Geometry check sheet. Reference: the model listing, model coordinates, mm. A direction names the side the tool comes from. Give positions to 0.01 mm unless a question says otherwise; leave off trailing zeros. Write each loop counter-clockwise with the first axis right and the second up, starting at its lowest first coordinate (ties: lowest second). Pieces come first, ordered by that corner, then holes. Notation, with made-up numbers: M -39.5,41.25 L -26.5,41.25 A18 cw -26.5,50.25 Z; hole C 64,44.5 d5. An arc over 180 degrees is marked long. One line per item, written item: value. Start each with the question number.
1. Cross-section at A-A on z = 0.6. Record the cut outline in (x, y), then the cut area to 3 significant figures.
2. Tool access check on faces 4 (the face through (6.7, 9.04, 2.96)), 5 (the face through (12, 3.25, 3)), 6 (the face through (4, -5, 5)). Record the directions out of +Z, -Z, +X, -X, +Y, -Y that give a thin tool (end or side, any length) a straight path to the whole face; none if there is none.
3. Release check for a two-part mould opening along Y. For faces 1 (the face through (0, -2, 1)), 2 (the face through (13, 4.23, 2.96)), 3 (the face through (-4.285, -10.949, 5.26)) record: pulls with the +Y half, pulls with the -Y half, needs draft (parallel to the pull), parting line crosses it, or undercut.
4. Cross-section at D-D on x = -5.75. Record the cut outline in (y, z), then the cut area to 3 significant figures.
5. Cross-section at B-B on y = -5.25. Record the cut outline in (x, z).
6. Cross-section at C-C on z = 1.9. Record the cut outline in (x, y), then the cut area to 3 significant figures.
7. Gauge pin test, flat ends, axial feed: pin 1 (1.6 mm diameter, centred on y = -7, z = 5.5, fed in from +X); pin 2 (1.5 mm diameter, centred on x = -2, z = 2.5, fed in from +Y); pin 3 (1.2 mm diameter, centred on x = -12, z = 2.5, fed in from -Y). Record the tip position at first contact, or that the pin passes through.
8. Scan lines: line 1 (Y direction, x = 0, z = 0.4); line 2 (Z direction, x = 11, y = -1.25); line 3 (Z direction, x = -1.5, y = -9.5). Record each from-to range of solid material in increasing order.
from build123d import *

# Parameters (mm, degrees)
F1_DEPTH  = 6
F2_T      = -1.5
F3_DEPTH  = 5
F4_T      = -1.5
F5_W      = 25.7072905079
F5_H      = 3
F6_DEPTH  = 14.5
F8_DEPTH  = 2
F9_R      = 2
F10_DEPTH = 25
F11_R     = 1
F12_R     = 1.5
F13_DEPTH = 2


with BuildPart() as f1:
    # F0 (on Top) → F1 (new body)
    with BuildSketch(Plane.XY):
        Polygon((8.1736034401, -11.25), (13.2251681766, 4.2971176266), (0, 13.9057647469), (-13.2251681766, 4.2971176266), (-8.1736034401, -11.25), align=None)
    extrude(amount=F1_DEPTH)

    # F2
    f2_openings = [f1.faces().sort_by_distance(p)[0] for p in [
        (10.699386, -3.476441, 3),
    ]]
    offset(amount=F2_T, openings=f2_openings)

    # F0 (on Top) → F3 (join)
    with BuildSketch(Plane.XY):
        Polygon((8.1736034401, -11.25), (13.2251681766, 4.2971176266), (0, 13.9057647469), (-13.2251681766, 4.2971176266), (-8.1736034401, -11.25), align=None)
    extrude(amount=F3_DEPTH)

    # F4
    f4_openings = [f1.faces().sort_by_distance(p)[0] for p in [
        (0, -11.25, 3),
    ]]
    offset(amount=F4_T, openings=f4_openings)

    # F5 (on face) → F6 (cut)
    with BuildSketch(Plane.XZ.offset(11.25)):
        with Locations((-0.012323726, 3)):
            Rectangle(F5_W, F5_H)
    extrude(amount=-F6_DEPTH, mode=Mode.SUBTRACT)

    # F7 (on face) → F8 (cut)
    with BuildSketch(Plane.XY.offset(6)):
        with BuildLine():
            Line((4, -12.5590292737), (4, 0))
            ThreePointArc((4, 0), (0, 4), (-4, 0))
            Line((-4, 0), (-4, -12.5590292737))
            Line((-4, -12.5590292737), (4, -12.5590292737))
        make_face()
    extrude(amount=-F8_DEPTH, mode=Mode.SUBTRACT)

    # F9 (on face) → F10 (cut)
    with BuildSketch(Plane.XY.offset(1.5)):
        Circle(F9_R)
    extrude(amount=-F10_DEPTH, mode=Mode.SUBTRACT)

    # F11
    f11_edges = [f1.edges().sort_by_distance(p)[0] for p in [
        (8.173603, -11.25, 5.25),
        (13.225168, 4.297118, 3),
        (8.173603, -11.25, 0.75),
        (-8.173603, -11.25, 0.75),
        (-8.173603, -11.25, 5.25),
        (-4, -11.25, 5.25),
        (4, -11.25, 5.25),
        (0, 13.905765, 3),
        (-13.225168, 4.297118, 3),
    ]]
    fillet(f11_edges, radius=F11_R)

    # F12 (on face) → F13 (cut)
    with BuildSketch(Plane.XY.offset(6)):
        with Locations((0, 8.8348483847)):
            Circle(F12_R)
    extrude(amount=-F13_DEPTH, mode=Mode.SUBTRACT)


solid = f1.part
Report:
1. outline: M -13,3.61 L -8.4,-10.56 A1 ccw -7.45,-11.25 L 7.45,-11.25 A1 ccw 8.4,-10.56 L 13,3.61 A1 ccw 12.64,4.72 L 0.59,13.48 A1 ccw -0.59,13.48 L -12.64,4.72 A1 ccw Z; hole C 0,0 d4
1. area: 447 mm^2
2. face 4: +Z, -Z, +X, +Y
2. face 5: -Y
2. face 6: +Z, -Y
3. face 1: undercut
3. face 2: parting line crosses it
3. face 3: pulls with the -Y half
4. outline: M -11.25,0 L 9.73,0 L 9.73,6 L -11.25,6 L -11.25,4.5 L 7.87,4.5 L 7.87,1.5 L -11.25,1.5 Z
4. area: 68.5 mm^2
5. outline: M -10.12,0 L 10.12,0 L 10.12,1.5 L -10.12,1.5 Z; M -10.12,4.5 L -4,4.5 L -4,6 L -10.12,6 Z; M 4,4.5 L 10.12,4.5 L 10.12,6 L 4,6 Z
6. outline: M -13,3.61 L -12.87,3.19 L -12.87,3.25 L -11.31,3.25 L -11.46,3.72 L 0,12.05 L 11.46,3.72 L 11.31,3.25 L 12.84,3.25 L 12.84,3.12 L 13,3.61 A1 ccw 12.64,4.72 L 0.59,13.48 A1 ccw -0.59,13.48 L -12.64,4.72 A1 ccw Z
6. area: 47.9 mm^2
7. pin 1: stops at x = 9.81
7. pin 2: stops at y = 13
7. pin 3: stops at y = 3.25
8. line 1: y = -11.25 to -2, 2 to 13.67
8. line 2: z = 0 to 1.5, 4.5 to 6
8. line 3: z = 0 to 1.5
